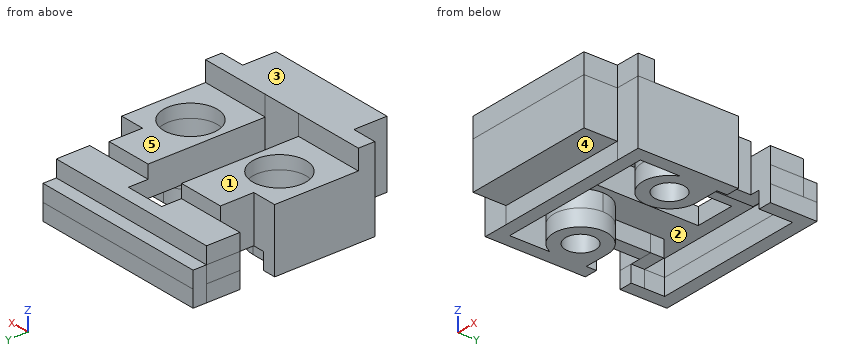
Autodesk Fusion 360 part; units mm, degrees
sketch "Sketch1" plane through (0, 0, 0) normal (0, 0, 1) x (1, 0, 0) in component "PecaPorta"
  line L0 (-37.704, -20.0025) -> (-33.9529, -19.9954)
  line L1 (-33.9529, -19.9954) -> (-33.9623, -14.9954)
  line L2 (-33.9623, -14.9954) -> (-37.4642, -15.002)
  line L3 (-37.4642, -15.002) -> (-37.4736, -10.0032)
  line L4 (-37.704, -20.0025) -> (-37.6758, -35.0025)
  line L5 (-10.4698, -9.9525) -> (-10.4604, -14.9513)
  line L6 (-10.1737, -34.9508) -> (-10.2018, -19.9508)
  line L7 (-10.2018, -19.9508) -> (-13.9529, -19.9579)
  line L8 (-13.9529, -19.9579) -> (-13.9623, -14.9579)
  line L9 (-10.4604, -14.9513) -> (-13.9623, -14.9579)
  line L10 (-26.9294, -32.5252) -> (-20.9294, -32.514)
  line L11 (-20.9294, -32.514) -> (-20.9679, -12.014)
  line L12 (-20.9679, -12.014) -> (-26.9679, -12.0253)
  line L13 (-26.9679, -12.0253) -> (-26.9294, -32.5252)
  circle A0 centre (-31.9407, -25.5003) radius 4
  circle A1 centre (-15.9407, -25.4703) radius 4
  line L14 (-33.9154, -39.9508) -> (-13.9154, -39.9508)
  line L15 (-33.9154, -39.9508) -> (-33.9247, -34.9954)
  line L16 (-13.9154, -39.9508) -> (-13.9248, -34.9579)
  line L17 (-10.4698, -9.9525) -> (-37.4736, -10.0032)
  circle A2 centre (-31.9407, -25.5003) radius 2.25
  circle A3 centre (-15.9407, -25.4703) radius 2.25
  line L18 (-10.4736, -7.9525) -> (-10.4698, -9.9525)
  line L19 (-10.4736, -7.9525) -> (-37.4736, -8.0032)
  line L20 (-37.4736, -8.0032) -> (-37.4736, -10.0032)
  line L21 (-37.6758, -35.0025) -> (-33.9247, -34.9954)
  line L22 (-13.9248, -34.9579) -> (-10.1737, -34.9508)
  line L23 (-13.9248, -34.9579) -> (-33.9247, -34.9954)
  line L24 (-12.1877, -32.9568) -> (-12.1991, -26.8848)
  line L25 (-12.2045, -24.0418) -> (-12.2084, -21.9579)
  line L26 (-12.2084, -21.9579) -> (-14.0206, -21.9613)
  line L27 (-15.9576, -12.9546) -> (-15.9416, -21.4703)
  line L28 (-15.9576, -12.9546) -> (-12.4668, -12.9481)
  line L29 (-12.4668, -12.9481) -> (-12.4724, -9.9562)
  line L30 (-12.1877, -32.9568) -> (-35.6814, -33.0009)
  line L31 (-35.6814, -33.0009) -> (-35.6929, -26.8864)
  line L32 (-35.6981, -24.1284) -> (-35.7021, -21.9994)
  line L33 (-33.8756, -21.9994) -> (-35.7021, -21.9994)
  line L34 (-31.9576, -21.5004) -> (-31.9736, -12.9987)
  line L35 (-31.9736, -12.9987) -> (-35.4689, -12.9987)
  line L36 (-35.4689, -12.9987) -> (-35.4745, -9.9994)
  line L37 (-13.9623, -14.9579) -> (-20.9623, -14.971)
  line L38 (-33.9623, -14.9954) -> (-26.9623, -14.9823)
  dimension "d28" = 20
  dimension "d40" = 27
extrude "Extrude7" add sketch "Sketch1" along normal blind 2.5 contours L0 L1 L4 L6 L7 L8 A0 A1 L21 L22 L23 L24 L25 L26 L27 L30 L31 L32 L33 L34 L37 L38 | L2 L3 L17 L34 L35 L36 L38 | L14 L15 L16 L23 | L10 L11 L13 A0 A1 L24 L27 L30 L31 L34 L37 L38 | L11 L12 L13 L17 L27 L28 L29 L34 L35 L36 L37 L38 | A0 L32 L33 | L5 L9 L17 L27 L28 L29 L37 | A1 L25 L26
sketch "Sketch3" plane through (0, 0, 2.5) normal (0, 0, 1) x (-1, 0, 0)
  circle A0 centre (31.9407, 25.5003) radius 4
  line L0 (26.9294, 32.5252) -> (26.9679, 12.0253)
  line L1 (26.9679, 12.0253) -> (20.9679, 12.014)
  line L2 (20.9679, 12.014) -> (20.9294, 32.514)
  line L3 (20.9294, 32.514) -> (26.9294, 32.5252)
  circle A1 centre (15.9407, 25.4703) radius 4
  line L4 (33.9154, 39.9508) -> (13.9154, 39.9508)
  line L5 (13.9154, 39.9508) -> (13.9248, 34.9579)
  line L6 (13.9248, 34.9579) -> (10.1737, 34.9508)
  line L7 (10.1737, 34.9508) -> (10.2018, 19.9508)
  line L8 (10.2018, 19.9508) -> (13.9529, 19.9579)
  line L9 (13.9529, 19.9579) -> (13.9623, 14.9579)
  line L10 (13.9623, 14.9579) -> (10.4604, 14.9513)
  line L11 (10.4604, 14.9513) -> (10.4698, 9.9525)
  line L12 (10.4698, 9.9525) -> (37.4736, 10.0032)
  line L13 (37.4736, 10.0032) -> (37.4642, 15.002)
  line L14 (37.4642, 15.002) -> (33.9623, 14.9954)
  line L15 (33.9623, 14.9954) -> (33.9529, 19.9954)
  line L16 (33.9529, 19.9954) -> (37.704, 20.0025)
  line L17 (37.704, 20.0025) -> (37.6758, 35.0025)
  line L18 (37.6758, 35.0025) -> (33.9247, 34.9954)
  line L19 (33.9247, 34.9954) -> (33.9154, 39.9508)
  line L20 (13.9623, 14.9579) -> (20.9623, 14.971)
  line L21 (33.9623, 14.9954) -> (26.9623, 14.9823)
  point P0 (20.9623, 14.971)
  point P1 (26.9623, 14.9823)
extrude "Extrude8" add sketch "Sketch3" along normal blind 2 contours L0 L2 L3 L4 L5 L6 L7 L8 L9 L15 L16 L17 L18 L19 L20 L21
extrude "Extrude9" add sketch "Sketch1" against normal blind 2.5 contours L0 L1 L4 L6 L7 L8 A0 A1 L21 L22 L23 L24 L25 L26 L27 L30 L31 L32 L33 L34 L37 L38 | L2 L3 L17 L34 L35 L36 L38 | L14 L15 L16 L23 | L17 L18 L19 L20 | A0 | A0 L32 L33 | L5 L9 L17 L27 L28 L29 L37 | A1 | A1 L25 L26
sketch "Sketch4" plane through (0, 0, -2.5) normal (0, 0, -1) x (1, 0, 0)
  circle A0 centre (-31.9407, 25.5003) radius 2.25
  line L0 (-12.1877, 32.9568) -> (-12.1991, 26.8848)
  arc A1 (-12.1991, 26.8848) -> (-15.9416, 21.4703) centre (-15.9407, 25.4703) ccw
  line L1 (-15.9416, 21.4703) -> (-15.9576, 12.9546)
  line L2 (-15.9576, 12.9546) -> (-12.4668, 12.9481)
  line L3 (-12.4668, 12.9481) -> (-12.4724, 9.9562)
  line L4 (-12.4724, 9.9562) -> (-35.4745, 9.9994)
  line L5 (-35.4745, 9.9994) -> (-35.4689, 12.9987)
  line L6 (-35.4689, 12.9987) -> (-31.9736, 12.9987)
  line L7 (-31.9736, 12.9987) -> (-31.9576, 21.5004)
  arc A2 (-31.9576, 21.5004) -> (-35.6929, 26.8864) centre (-31.9407, 25.5003) ccw
  line L8 (-35.6929, 26.8864) -> (-35.6814, 33.0009)
  line L9 (-35.6814, 33.0009) -> (-12.1877, 32.9568)
  circle A3 centre (-15.9407, 25.4703) radius 2.25
  line L10 (-13.9154, 39.9508) -> (-33.9154, 39.9508)
  line L11 (-33.9154, 39.9508) -> (-33.9247, 34.9954)
  line L12 (-33.9247, 34.9954) -> (-37.6758, 35.0025)
  line L13 (-37.6758, 35.0025) -> (-37.704, 20.0025)
  line L14 (-37.704, 20.0025) -> (-33.9529, 19.9954)
  line L15 (-33.9529, 19.9954) -> (-33.9623, 14.9954)
  line L16 (-33.9623, 14.9954) -> (-37.4642, 15.002)
  line L17 (-37.4642, 15.002) -> (-37.4736, 10.0032)
  line L18 (-37.4736, 10.0032) -> (-37.4736, 8.0032)
  line L19 (-37.4736, 8.0032) -> (-10.4736, 7.9525)
  line L20 (-10.4736, 7.9525) -> (-10.4604, 14.9513)
  line L21 (-10.4604, 14.9513) -> (-13.9623, 14.9579)
  line L22 (-13.9623, 14.9579) -> (-13.9529, 19.9579)
  line L23 (-13.9529, 19.9579) -> (-10.2018, 19.9508)
  line L24 (-10.2018, 19.9508) -> (-10.1737, 34.9508)
  line L25 (-10.1737, 34.9508) -> (-13.9248, 34.9579)
  line L26 (-13.9248, 34.9579) -> (-13.9154, 39.9508)
  line L27 (-35.4689, 12.9987) -> (-35.4651, 14.9983)
  line L28 (-33.9247, 34.9954) -> (-13.9248, 34.9579)
  line L29 (-12.4668, 12.9481) -> (-12.463, 14.9551)
  circle A4 centre (-15.9407, 25.4703) radius 4
  circle A5 centre (-31.9407, 25.5003) radius 4
  line L30 (-15.9416, 21.4703) -> (-12.2093, 21.4694)
  line L31 (-12.2093, 21.4694) -> (-12.2122, 19.9546)
  line L32 (-31.9576, 21.5004) -> (-35.703, 21.5162)
  line L33 (-35.703, 21.5162) -> (-35.7058, 19.9987)
extrude "Extrude10" add sketch "Sketch4" along normal blind 2.5 contours L0 L8 L9 L12 L13 L14 L23 L24 L25 L28 A4 A5 L30 L31 L32 L33 | A1 A4 | A2 A5 | L3 L4 L5 L16 L17 L18 L19 L20 L21 L27 L29
sketch "Sketch5" plane through (0, 0, 4.5) normal (0, 0, 1) x (-1, 0, 0)
  circle A0 centre (15.9407, 25.4703) radius 4
  circle A1 centre (31.9407, 25.5003) radius 4
  line L0 (33.9529, 19.9954) -> (37.704, 20.0025)
  line L1 (37.704, 20.0025) -> (37.6758, 35.0025)
  line L2 (37.6758, 35.0025) -> (33.9247, 34.9954)
  line L3 (33.9247, 34.9954) -> (33.9154, 39.9508)
  line L4 (33.9154, 39.9508) -> (13.9154, 39.9508)
  line L5 (13.9154, 39.9508) -> (13.9248, 34.9579)
  line L6 (13.9248, 34.9579) -> (10.1737, 34.9508)
  line L7 (10.1737, 34.9508) -> (10.2018, 19.9508)
  line L8 (10.2018, 19.9508) -> (13.9529, 19.9579)
  line L9 (13.9529, 19.9579) -> (13.9623, 14.9579)
  line L10 (13.9623, 14.9579) -> (20.9623, 14.971)
  line L11 (20.9623, 14.971) -> (20.9294, 32.514)
  line L12 (20.9294, 32.514) -> (26.9294, 32.5252)
  line L13 (26.9294, 32.5252) -> (26.9623, 14.9823)
  line L14 (26.9623, 14.9823) -> (33.9623, 14.9954)
  line L15 (33.9623, 14.9954) -> (33.9529, 19.9954)
  line L16 (20.9294, 32.514) -> (10.1783, 32.4938)
  line L17 (26.9294, 32.5252) -> (37.6805, 32.5454)
extrude "Extrude11" add sketch "Sketch5" along normal blind 3 contours L1 L2 L3 L4 L5 L6 L7 L12 L16 L17
component "PecaPorta" placed x (1, 0, 0) y (0, 1, 0) z (0, 0, 1) at (0, 0, 0)
Work out the finished part from the listing and answer in its coordinate system (mm). Face numbers are marked on the shaded views. A direction names the side the tool comes from. Coordinates: 2 decimals unless noted, no trailing zeros. Write each loop counter-clockwise with the first axis right and the second up, starting at its lowest first coordinate (ties: lowest second). Pieces come first, ordered by that corner, then holes.
Q1. Find the intervals of material crossed by line 1 (Y direction, x = -13, z = -0.25); line 2 (X direction, y = -18.5, z = 3.5); line 3 (Y direction, x = -15.5, z = -1), in increasing order.
Q2. Which of the six approach directions +Z, -Z, +X, -X, +Y, -Y give full straight-line access (tool end or side, diameter ignored) to the marked faces 3, 4 and 5?
Q3. Each of these flat-tipped pins is pushed along its axis until it touches: pin 1 Ø5.5 at (x, y) = (-31, -24) entering from +Z; pin 2 Ø1.2 at (x, z) = (-33, -1) entering from +Y; pin 3 Ø1.1 at (x, y) = (-34, -18.5) entering from -Z; pin 4 Ø2 at (x, y) = (-22, -19.5) entering from -Z. Where does it stop, or does it pass through?
Q4. A cutting plane is placed at A-A, the plane y = -20.5. Give the vertices of the cut face in (x, z), then the cut area to 3 significant figures.
Q5. A cutting plane is placed at D-D, the plane z = 1.25. Give the vertices of the cut face in (x, y).
Q6. Determine the mould class of the marked faces 1 and 2 for opening direction Y: released by +Y, released by -Y, zero draft, split by the parting line, or undercut.
Findings below:
1. line 1: y = -34.96 to -32.96, -28.18 to -19.96, -14.96 to -12.95, -9.96 to -7.96
1. line 2: x = -33.96 to -26.96, -20.96 to -13.96
1. line 3: y = -39.95 to -32.96, -29.45 to -27.68, -23.26 to -12.95, -9.96 to -7.96
2. face 3: +Z, +X, -X, +Y, -Y
2. face 4: -Z, +X, -X, -Y
2. face 5: +Z, +X, -X, +Y
3. pin 1: stops at z = 4.5
3. pin 2: stops at y = -7.99
3. pin 3: stops at z = -2.5
3. pin 4: passes through
4. outline: (-37.7, -5) - (-35.7, -5) - (-35.7, -2.5) - (-31.96, -2.5) - (-31.96, 0) - (-26.95, 0) - (-26.95, 4.5) - (-37.7, 4.5) - close; (-20.95, 0) - (-15.94, 0) - (-15.94, -2.5) - (-12.21, -2.5) - (-12.21, -5) - (-10.2, -5) - (-10.2, 4.5) - (-20.95, 4.5) - close
4. area: 135 mm2
5. outline: (-37.7, -20) - (-37.68, -35) - (-33.92, -35) - (-33.92, -39.95) - (-13.92, -39.95) - (-13.92, -34.96) - (-10.17, -34.95) - (-10.2, -19.95) - (-13.95, -19.96) - (-13.96, -14.96) - (-10.46, -14.95) - (-10.47, -9.95) - (-37.47, -10) - (-37.46, -15) - (-33.96, -15) - (-33.95, -20) - close; hole circle Ø8 at (-31.94, -25.5); hole (-26.97, -12.03) - (-26.93, -32.53) - (-20.93, -32.51) - (-20.97, -12.01) - close; hole circle Ø8 at (-15.94, -25.47)
6. face 1: zero draft
6. face 2: undercut
